Check sheet for the modelled part. Datum: model origin and axes. Units: mm. Coordinates: 2 decimals unless noted, no trailing zeros. Order: outer loops, then holes, each group sorted by start corner. A loop starts at its lowest first (then second) coordinate and runs counter-clockwise, first axis right, second up.
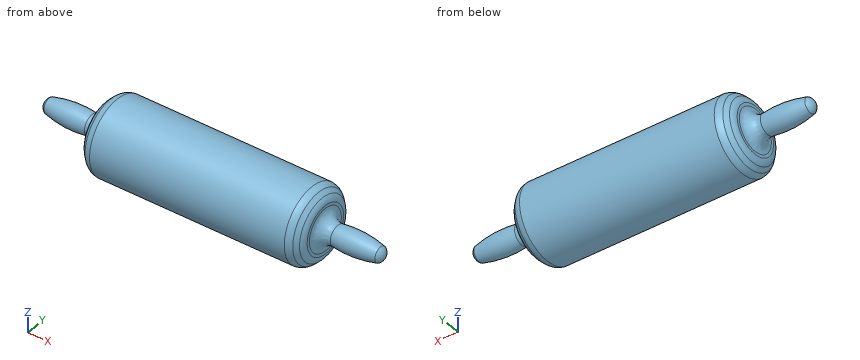
from build123d import *

# Parameters (mm, degrees)
F2_SIZE = 6.35
F3_R    = 6.35
F4_R    = 7.62


with BuildPart() as f1:
    # F0 (on Front) → F1 (revolve)
    with BuildSketch(Plane.XZ):
        with BuildLine():
            Line((-113.4249120951, 0), (-78.4026022691, 0))
            Line((-78.4026022691, 0), (73.9973977309, 0))
            Line((73.9973977309, 0), (109.0197075568, 0))
            Line((109.0197075568, 0), (115.0176400335, 0))
            ThreePointArc((115.0176400335, 0), (114.2367455979, 2.9593425069), (112.0973977309, 5.1481081173))
            ThreePointArc((112.0973977309, 5.1481081173), (93.0473977309, 7.6165926694), (73.9973977309, 5.1481081173))
            Line((73.9973977309, 5.1481081173), (73.9973977309, 25.4))
            Line((73.9973977309, 25.4), (-78.4026022691, 25.4))
            Line((-78.4026022691, 25.4), (-78.4026022691, 5.1481081173))
            ThreePointArc((-78.4026022691, 5.1481081173), (-97.4526022691, 7.6165926694), (-116.5026022691, 5.1481081173))
            ThreePointArc((-116.5026022691, 5.1481081173), (-118.6419501361, 2.9593425069), (-119.4228445717, 0))
            Line((-119.4228445717, 0), (-113.4249120951, 0))
        make_face()
    revolve(axis=Axis((-2.2026022691, 0, 0), (1, 0, 0)))

    # F2
    f2_edges = [f1.edges().sort_by_distance(p)[0] for p in [
        (73.997398, 0, -25.4),
        (-78.402602, 0, -25.4),
    ]]
    chamfer(f2_edges, length=F2_SIZE)

    # F3
    f3_edges = [f1.edges().sort_by_distance(p)[0] for p in [
        (73.997398, 0, -19.05),
        (67.647398, 0, -25.4),
        (-78.402602, 0, -19.05),
        (-72.052602, 0, -25.4),
    ]]
    fillet(f3_edges, radius=F3_R)

    # F4
    f4_edges = [f1.edges().sort_by_distance(p)[0] for p in [
        (73.997398, 0, -5.148108),
        (-78.402602, 0, -5.148108),
    ]]
    fillet(f4_edges, radius=F4_R)


solid = f1.part
(1) Cross-section at A-A (x = 29). Enter the section's corners in (y, z).
Filled in:
outline: circle Ø50.8 at (0, 0)
(2) Go/stop test with flat-tipped pins: P1, Ø10, axis at x = -32, y = 16, coming from the +Z side; P2, Ø5, axis at x = 57.5, z = -12.5, coming from the +Y side; P3, Ø12, axis at x = -69.5, y = -12, coming from the +Z side. Record where each tip stops, or that it passes through.
Filled in:
P1: stops at z = 22.89
P2: stops at y = 23.35
P3: stops at z = 24.68
(3) Thickness scan on probe 1 along X at (y, z) = (11.5, -10.5); probe 2 along X at (y, z) = (-4, -2); probe 3 along Y at (x, z) = (5, 10.5). Record the ranges inside material, lowest first.
Filled in:
probe 1: x = -78.4 to 74
probe 2: x = -117.42 to 113.02
probe 3: y = -23.13 to 23.13
